```python
from build123d import *

# Parameters (mm, degrees)
PAD012_DEPTH    = 4
PAD013_DEPTH    = 45
PAD014_DEPTH    = 2
SKETCH043_R     = 20
POCKET021_DEPTH = 6
SKETCH044_R     = 24
POCKET022_DEPTH = 2
SKETCH052_R     = 2
POCKET025_DEPTH = 2
SKETCH053_R     = 1
POCKET026_DEPTH = 2


with BuildPart() as part:
    # Sketch036 (on Face1 of CopyPad006) → Pad012 (new body)
    with BuildSketch(Plane.XY.offset(58)):
        with BuildLine():
            Line((0, -50), (50, -50))
            Line((50, -50), (50, 30))
            Line((50, 30), (-50, 30))
            Line((-50, 30), (-50, 0))
            ThreePointArc((-50, 0), (-35.3553390593, -35.3553390593), (0, -50))
        make_face()
    extrude(amount=PAD012_DEPTH)

    # Sketch037 (on Face6 of Pad012) → Pad013 (join)
    with BuildSketch(Plane(origin=(0, 0, 58), x_dir=(1, 0, 0), z_dir=(0, 0, -1))):
        with BuildLine():
            ThreePointArc((0, 26), (-18.3847763109, 18.3847763108), (-26, 0))
            Line((-26, -15), (-26, 0))
            Line((-24, -15), (-26, -15))
            Line((-24, 0), (-24, -15))
            ThreePointArc((0, 24), (-16.9705627485, 16.9705627485), (-24, 0))
            Line((0, 24), (15, 24))
            Line((15, 24), (15, 26))
            Line((15, 26), (0, 26))
        make_face()
    extrude(amount=PAD013_DEPTH)

    # Sketch038 (on Face4 of Pad013) → Pad014 (join)
    with BuildSketch(Plane(origin=(0, 0, 58), x_dir=(1, 0, 0), z_dir=(0, 0, -1))):
        with BuildLine():
            Line((0, 46), (46, 46))
            Line((46, 46), (46, -26))
            Line((46, -26), (-46, -26))
            Line((-46, -26), (-46, 0))
            ThreePointArc((0, 46), (-32.5269119346, 32.5269119346), (-46, 0))
        make_face()
    extrude(amount=PAD014_DEPTH)

    # Sketch043 (on Face5 of Pad014) → Pocket021 (cut)
    with BuildSketch(Plane.XY.offset(62)):
        Circle(SKETCH043_R)
    extrude(amount=-POCKET021_DEPTH, mode=Mode.SUBTRACT)

    # Sketch044 (on Face5 of Pocket021) → Pocket022 (cut)
    with BuildSketch(Plane.XY.offset(62)):
        Circle(SKETCH044_R)
    extrude(amount=-POCKET022_DEPTH, mode=Mode.SUBTRACT)

    # Sketch052 (on Face5 of Pocket022) → Pocket025 (cut)
    with BuildSketch(Plane.XY.offset(62)):
        with Locations((-47.7, 27.7)):
            Circle(SKETCH052_R)
        with Locations((47.7, 27.7)):
            Circle(SKETCH052_R)
        with Locations((47.7, -47.71)):
            Circle(SKETCH052_R)
    extrude(amount=-POCKET025_DEPTH, mode=Mode.SUBTRACT)

    # Sketch053 (on Face21 of Pocket025) → Pocket026 (cut)
    with BuildSketch(Plane.XY.offset(60)):
        with Locations((-47.7, 27.7)):
            Circle(SKETCH053_R)
        with Locations((47.7, 27.7)):
            Circle(SKETCH053_R)
        with Locations((47.7, -47.71)):
            Circle(SKETCH053_R)
    extrude(amount=-POCKET026_DEPTH, mode=Mode.SUBTRACT)


solid = part.part
```
Can you work these out from the model? Positions are in its coordinate system, mm. A direction names the side the tool comes from. Round coordinates to 2 decimals unless told otherwise and drop trailing zeros. Loops run counter-clockwise (first coordinate to the right, second up) from the corner with the lowest first, then second, coordinate; pieces in that order, holes last. Notation, with made-up numbers: M 81.25,-36.5 L 85.25,-36.5 A17 ccw 85.25,-30.5 Z; hole C 7,-25 d1. An arc over 180 degrees is marked long. Answer in a Markdown table with one row per item.
1. On a 3-axis mill with a long thin cutter (end or side, diameter ignored), from which of +Z, -Z, +X, -X, +Y, -Y can I reach the whole of each face in a straight line? I mean faces 4 (the face through (-26, 8, 35)), 5 (the face through (-32.17, -32.88, 57.01)), 6 (the face through (45.702, 27.788, 61.014)). Say none if no direction works.
Established:
| item | result |
|---|---|
| face 4 | -Z, -X, +Y, -Y |
| face 5 | -Z, -X, -Y |
| face 6 | +Z |
2. If we section it at D-D, the plane y = -40.5: Please give me the cut outline in (x, z), plus the area to 3 significant figures.
Established:
| item | result |
|---|---|
| outline | M -29.32,58 L -21.81,58 L -21.81,56 L 46,56 L 46,58 L 50,58 L 50,62 L -29.32,62 Z |
| area | 453 mm² |
3. Please list where these lines run through material, in increasing order: line 1 (Y direction, x = 47.7, z = 58.6); line 2 (X direction, y = 27, z = 59); line 3 (Z direction, x = 43, y = -34.5). Write a range as from..to.
Established:
| item | result |
|---|---|
| line 1 | -50..-48.71, -46.71..26.7, 28.7..30 |
| line 2 | -50..-48.41, -46.99..46.99, 48.41..50 |
| line 3 | 56..62 |
4. If we section it at C-C, the plane y = -12: Please give me the cut outline in (x, z), plus the area to 3 significant figures.
Established:
| item | result |
|---|---|
| outline | M -48.54,58 L -44.41,58 L -44.41,56 L -23.07,56 L -23.07,13 L -20.78,13 L -20.78,56 L -16,56 L -16,60 L -20.78,60 L -20.78,62 L -48.54,62 Z; M 16,56 L 46,56 L 46,58 L 50,58 L 50,62 L 20.78,62 L 20.78,60 L 16,60 Z |
| area | 462 mm² |
5. I'm going to push flat-ended pins straight in: pin 1 Ø2.5 at (x, y) = (47.7, -47.71) entering from -Z; pin 2 Ø2 at (x, y) = (47.5, -47.5) entering from +Z; pin 3 Ø7.5 at (x, z) = (8.5, 28.5) entering from +Y; pin 4 Ø1 at (x, z) = (17, 44) entering from -Y. Where does each tip first touch, or does it pass through?
Established:
| item | result |
|---|---|
| pin 1 | z = 58 |
| pin 2 | z = 60 |
| pin 3 | y = -24 |
| pin 4 | through |
6. If we section it at B-B, the plane x = -10.5: Please give me the cut outline in (y, z), plus the area to 3 significant figures.
Established:
| item | result |
|---|---|
| outline | M -48.89,58 L -44.79,58 L -44.79,56 L -23.79,56 L -23.79,13 L -21.58,13 L -21.58,56 L -17.02,56 L -17.02,60 L -21.58,60 L -21.58,62 L -48.89,62 Z; M 17.02,56 L 26,56 L 26,58 L 30,58 L 30,62 L 21.58,62 L 21.58,60 L 17.02,60 Z |
| area | 329 mm² |
7. If we section it at A-A, the plane z = 24: Please give me the cut outline in (x, y), plus the area to 3 significant figures.
Established:
| item | result |
|---|---|
| outline | M -26,0 A26 ccw 0,-26 L 15,-26 L 15,-24 L 0,-24 A24 cw -24,0 L -24,15 L -26,15 Z |
| area | 139 mm² |
8. Thinking about a two-plate mould opening in Y: for faces 1 (the face through (-19, -15, 13)), 2 (the face through (-45.853, 26.934, 61.014)), 3 (the face through (7, -24, 35)), which applies, pulls with the +Y half, pulls with the -Y half, needs draft (parallel to the pull), parting line crosses it, or undercut?
Established:
| item | result |
|---|---|
| face 1 | needs draft |
| face 2 | undercut |
| face 3 | pulls with the +Y half |
